Can you work these out from the model? Positions are in its coordinate system, mm. Face numbers are marked on the shaded views. A direction names the side the tool comes from. Coordinates: 2 decimals unless noted, no trailing zeros. Loops run counter-clockwise (first coordinate to the right, second up) from the corner with the lowest first, then second, coordinate; pieces in that order, holes last. Notation, with made-up numbers: (65, 62) -> (114, 62) arc R10 ccw to (114, 77) -> close; hole circle Ø4 at (66.5, 46.25). An arc over 180 degrees is marked (long way). Put each result on its own line as item: value. Start each with the question number.
Item 1: Will these pins go through, and if not, where does the flat tip stop? P1, Ø12, axis at x = 100, z = -27.5, coming from the +Y side; P2, Ø1, axis at y = 6, z = -17, coming from the -X side; P3, Ø1, axis at y = 1, z = -54.5, coming from the -X side.
Item 2: For the marked faces 1 and 2, which set-ups out of +Z, -Z, +X, -X, +Y, -Y let a thin tool reach every point of the face, with its end or its side?
Item 3: If we section it at B-B on z = -37: Please give me the cut outline in (x, y), plus the area to 3 significant figures.
Item 4: Please list where these lines run through material, in increasing order: L1, parallel to Y at x = 8, z = -27; L2, parallel to X at y = 7.5, z = -56; L3, parallel to X at y = 6.5, z = -65.5. Write a range as from..to.
Item 5: If we section it at A-A on x = 120.5: Please give me the cut outline in (y, z), plus the area to 3 significant figures.
```python
from build123d import *

# Parameters (mm, degrees)
ESQUISSE1_W             = 160
ESQUISSE1_H             = 80
BOSS_EXTRU_1_DEPTH      = 2
ENL_V_MAT_EXTRU_2_DEPTH = 2
ENL_V_MAT_EXTRU_3_DEPTH = 2
BOSS_EXTRU_2_DEPTH      = 6
ENL_V_MAT_EXTRU_4_REACH = 10
D_GAGEMENT_M21_D        = 2.4
D_GAGEMENT_M22_D        = 2.4
D_GAGEMENT_M23_D        = 2.4
D_GAGEMENT_M24_D        = 2.4


with BuildPart() as part:
    # Esquisse1 → Boss.-Extru.1 (new body)
    with BuildSketch(Plane(origin=(0, 0, 0), x_dir=(1, 0, 0), z_dir=(0, 1, 0))):
        with Locations((80, 40)):
            Rectangle(ESQUISSE1_W, ESQUISSE1_H)
    extrude(amount=BOSS_EXTRU_1_DEPTH)

    # Esquisse2 → Enlèv. mat.-Extru.2 (cut)
    with BuildSketch(Plane(origin=(0, 2, 0), x_dir=(1, 0, 0), z_dir=(0, 1, 0))):
        Polygon((0, 50), (30, 80), (0, 80), align=None)
        Polygon((130, 80), (160, 50), (160, 80), align=None)
        Polygon((130, 0), (160, 30), (160, 0), align=None)
        Polygon((0, 30), (30, 0), (0, 0), align=None)
    extrude(amount=-ENL_V_MAT_EXTRU_2_DEPTH, mode=Mode.SUBTRACT)

    # Esquisse7 → Enlèv. mat.-Extru.3 (cut)
    with BuildSketch(Plane(origin=(0, 2, 0), x_dir=(1, 0, 0), z_dir=(0, 1, 0))):
        with BuildLine():
            Line((62.95, 23), (62.95, 33))
            ThreePointArc((62.95, 33), (64, 34.05), (65.05, 33))
            Line((65.05, 33), (65.05, 23))
            ThreePointArc((65.05, 23), (64, 21.95), (62.95, 23))
        make_face()
        with BuildLine():
            Line((50.95, 23), (50.95, 33))
            ThreePointArc((50.95, 33), (52, 34.05), (53.05, 33))
            Line((53.05, 33), (53.05, 23))
            ThreePointArc((53.05, 23), (52, 21.95), (50.95, 23))
        make_face()
        with BuildLine():
            Line((50.95, 47), (50.95, 57))
            ThreePointArc((50.95, 57), (52, 58.05), (53.05, 57))
            Line((53.05, 57), (53.05, 47))
            ThreePointArc((53.05, 47), (52, 45.95), (50.95, 47))
        make_face()
        with BuildLine():
            Line((62.95, 47), (62.95, 57))
            ThreePointArc((62.95, 57), (64, 58.05), (65.05, 57))
            Line((65.05, 57), (65.05, 47))
            ThreePointArc((65.05, 47), (64, 45.95), (62.95, 47))
        make_face()
        with BuildLine():
            Line((97.05, 47), (97.05, 57))
            ThreePointArc((97.05, 57), (96, 58.05), (94.95, 57))
            Line((94.95, 57), (94.95, 47))
            ThreePointArc((94.95, 47), (96, 45.95), (97.05, 47))
        make_face()
        with BuildLine():
            Line((109.05, 47), (109.05, 57))
            ThreePointArc((109.05, 57), (108, 58.05), (106.95, 57))
            Line((106.95, 57), (106.95, 47))
            ThreePointArc((106.95, 47), (108, 45.95), (109.05, 47))
        make_face()
        with BuildLine():
            Line((109.05, 23), (109.05, 33))
            ThreePointArc((109.05, 33), (108, 34.05), (106.95, 33))
            Line((106.95, 33), (106.95, 23))
            ThreePointArc((106.95, 23), (108, 21.95), (109.05, 23))
        make_face()
        with BuildLine():
            Line((97.05, 23), (97.05, 33))
            ThreePointArc((97.05, 33), (96, 34.05), (94.95, 33))
            Line((94.95, 33), (94.95, 23))
            ThreePointArc((94.95, 23), (96, 21.95), (97.05, 23))
        make_face()
    extrude(amount=-ENL_V_MAT_EXTRU_3_DEPTH, mode=Mode.SUBTRACT)

    # Esquisse8 → Boss.-Extru.2 (add)
    with BuildSketch(Plane(origin=(0, 2, 0), x_dir=(1, 0, 0), z_dir=(0, 1, 0))):
        Polygon((13.029437252, 16.970562748), (19.393398282, 10.606601718), (33.535533906, 24.748737342), (27.171572875, 31.112698372), align=None)
        Polygon((19.393398282, 69.393398282), (13.029437252, 63.029437252), (27.171572875, 48.887301628), (33.535533906, 55.251262658), align=None)
        Polygon((149.393398282, 60.606601718), (143.029437252, 66.970562748), (128.887301628, 52.828427125), (135.251262658, 46.464466094), align=None)
        Polygon((146.970562748, 16.970562748), (140.606601718, 10.606601718), (126.464466094, 24.748737342), (132.828427125, 31.112698372), align=None)
    extrude(amount=BOSS_EXTRU_2_DEPTH)

    # Esquisse10 → Enlèv. mat.-Extru.4 (cut, up to next)
    with BuildSketch(Plane(origin=(0, 8, 0), x_dir=(1, 0, 0), z_dir=(0, 1, 0)), mode=Mode.PRIVATE) as enl_v_mat_extru_4_sk1:
        Polygon((17.97918472, 12.02081528), (14.443650814, 15.556349186), (28.585786438, 29.69848481), (32.121320344, 26.162950904), align=None)
    enl_v_mat_extru_4_tool1 = extrude(enl_v_mat_extru_4_sk1.sketch, amount=-ENL_V_MAT_EXTRU_4_REACH, mode=Mode.PRIVATE) & part.part
    add(enl_v_mat_extru_4_tool1.solids().sort_by_distance((23.282486, 8, -20.85965))[0], mode=Mode.SUBTRACT)
    # Esquisse10 → Enlèv. mat.-Extru.4 (cut, up to next)
    with BuildSketch(Plane(origin=(0, 8, 0), x_dir=(1, 0, 0), z_dir=(0, 1, 0)), mode=Mode.PRIVATE) as enl_v_mat_extru_4_sk2:
        Polygon((14.443650814, 64.443650814), (17.97918472, 67.97918472), (32.121320344, 53.837049096), (28.585786438, 50.30151519), align=None)
    enl_v_mat_extru_4_tool2 = extrude(enl_v_mat_extru_4_sk2.sketch, amount=-ENL_V_MAT_EXTRU_4_REACH, mode=Mode.PRIVATE) & part.part
    add(enl_v_mat_extru_4_tool2.solids().sort_by_distance((23.282486, 8, -59.14035))[0], mode=Mode.SUBTRACT)
    # Esquisse10 → Enlèv. mat.-Extru.4 (cut, up to next)
    with BuildSketch(Plane(origin=(0, 8, 0), x_dir=(1, 0, 0), z_dir=(0, 1, 0)), mode=Mode.PRIVATE) as enl_v_mat_extru_4_sk3:
        Polygon((144.443650814, 65.556349186), (147.97918472, 62.02081528), (133.837049096, 47.878679656), (130.30151519, 51.414213562), align=None)
    enl_v_mat_extru_4_tool3 = extrude(enl_v_mat_extru_4_sk3.sketch, amount=-ENL_V_MAT_EXTRU_4_REACH, mode=Mode.PRIVATE) & part.part
    add(enl_v_mat_extru_4_tool3.solids().sort_by_distance((139.14035, 8, -56.717514))[0], mode=Mode.SUBTRACT)
    # Esquisse10 → Enlèv. mat.-Extru.4 (cut, up to next)
    with BuildSketch(Plane(origin=(0, 8, 0), x_dir=(1, 0, 0), z_dir=(0, 1, 0)), mode=Mode.PRIVATE) as enl_v_mat_extru_4_sk4:
        Polygon((145.556349186, 15.556349186), (142.02081528, 12.02081528), (127.878679656, 26.162950904), (131.414213562, 29.69848481), align=None)
    enl_v_mat_extru_4_tool4 = extrude(enl_v_mat_extru_4_sk4.sketch, amount=-ENL_V_MAT_EXTRU_4_REACH, mode=Mode.PRIVATE) & part.part
    add(enl_v_mat_extru_4_tool4.solids().sort_by_distance((136.717514, 8, -20.85965))[0], mode=Mode.SUBTRACT)

    # Dégagement M21 (through all)
    with Locations(Plane(origin=(4.393398282, 0, 4.393398282), x_dir=(0.707106781, 0, -0.707106781), z_dir=(0.707106781, 0, 0.707106781))):
        with Locations((25.213203436, 5), (37.213203436, 5)):
            Hole(D_GAGEMENT_M21_D / 2)

    # Dégagement M22 (through all)
    with Locations(Plane(origin=(38.029437252, 0, -38.029437252), x_dir=(0.707106781, 0, 0.707106781), z_dir=(-0.707106781, 0, 0.707106781))):
        with Locations((-31.355339059, 5), (-19.355339059, 5)):
            Hole(D_GAGEMENT_M22_D / 2)

    # Dégagement M23 (through all)
    with Locations(Plane(origin=(75.606601718, 0, -75.606601718), x_dir=(0.707106781, 0, 0.707106781), z_dir=(-0.707106781, 0, 0.707106781))):
        with Locations((75.923881554, 5), (87.923881554, 5)):
            Hole(D_GAGEMENT_M23_D / 2)

    # Dégagement M24 (through all)
    with Locations(Plane(origin=(38.029437252, 0, 38.029437252), x_dir=(-0.707106781, 0, 0.707106781), z_dir=(-0.707106781, 0, -0.707106781))):
        with Locations((-144.492424049, 5), (-132.492424049, 5)):
            Hole(D_GAGEMENT_M24_D / 2)


solid = part.part
```
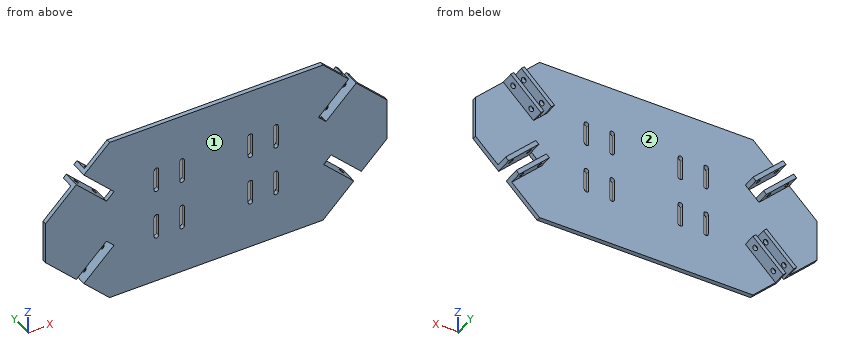
Solutions:
1. P1: y = 2
1. P2: x = 13.03
1. P3: x = 4
2. face 1: +Z, -Z, +X, -X, -Y
2. face 2: +Y
3. outline: (0, 0) -> (160, 0) -> (160, 2) -> (0, 2) -> close
3. area: 320 mm^2
4. L1: 0..2
4. L2: 20.06..22.89, 29.96..32.79, 132.06..134.89, 141.96..144.79
4. L3: 20.46..23.29, 141.56..144.39
5. outline: (0, -80) -> (2, -80) -> (2, 0) -> (0, 0) -> close
5. area: 160 mm^2
